from build123d import *

# Parameters (mm, degrees)
SKETCH1_R           = 1.5
SKETCH1_W           = 42
SKETCH1_H           = 20.5
BOSS_EXTRUDE1_DEPTH = 4


with BuildPart() as part:
    # Sketch1 → Boss-Extrude1 (new body)
    with BuildSketch(Plane.XY):
        with BuildLine():
            Line((0, 0), (0, 28))
            Line((0, 28), (-54, 28))
            Line((-54, 28), (-54, 33))
            Line((-54, 33), (-78, 33))
            Line((-78, 33), (-78, 28))
            Line((-78, 28), (-92, 28))
            Line((-92, 28), (-92, 21.4))
            Line((-92, 21.4), (-88, 21.4))
            ThreePointArc((-88, 21.4), (-86, 19.4), (-88, 17.4))
            Line((-88, 17.4), (-92, 17.4))
            Line((-92, 17.4), (-92, 11.6))
            Line((-92, 11.6), (-88, 11.6))
            ThreePointArc((-88, 11.6), (-86, 9.6), (-88, 7.6))
            Line((-88, 7.6), (-92, 7.6))
            Line((-92, 7.6), (-92, 0))
            Line((-92, 0), (0, 0))
        make_face()
        with Locations((-10, 21)):
            Circle(SKETCH1_R, mode=Mode.SUBTRACT)
        with Locations((-10, 6)):
            Circle(SKETCH1_R, mode=Mode.SUBTRACT)
        with Locations((-63, 14.5)):
            Rectangle(SKETCH1_W, SKETCH1_H, mode=Mode.SUBTRACT)
    extrude(amount=BOSS_EXTRUDE1_DEPTH)


solid = part.part
CAD build for the part. Positions are in the model's coordinates, mm. A direction names the side the tool comes from. Coordinates: 2 decimals unless noted, no trailing zeros. Order: outer loops, then holes, each group sorted by start corner. A loop starts at its lowest first (then second) coordinate and runs counter-clockwise, first axis right, second up.
Item 1: Band-saw the part on C-C on z = 2.3. List the corners of the cut face in (x, y).
Check sheet entries:
outline: (-92, 0) - (0, 0) - (0, 28) - (-54, 28) - (-54, 33) - (-78, 33) - (-78, 28) - (-92, 28) - (-92, 21.4) - (-88, 21.4) arc R2 cw to (-88, 17.4) - (-92, 17.4) - (-92, 11.6) - (-88, 11.6) arc R2 cw to (-88, 7.6) - (-92, 7.6) - close; hole (-84, 4.25) - (-42, 4.25) - (-42, 24.75) - (-84, 24.75) - close; hole circle Ø3 at (-10, 6); hole circle Ø3 at (-10, 21)
Item 2: Pin check, flat tips, straight feed: pin 1 Ø1.2 at (x, z) = (-89.5, 2.5) entering from +Y; pin 2 Ø2 at (y, z) = (30.5, 2.5) entering from -X; pin 3 Ø8 at (x, y) = (-69.5, 8.5) entering from -Z; pin 4 Ø2 at (y, z) = (10, 2.5) entering from -X. Stop position of each tip, or through.
Check sheet entries:
pin 1: stops at y = 28
pin 2: stops at x = -78
pin 3: passes through
pin 4: stops at x = -86.57
Item 3: 3-axis set-ups, long thin cutter, end or side, ignore diameter. For faces 1 (the face through (-90, 11.6, 2)), 2 (the face through (-36, 17, 0)), 3 (the face through (-27, 28, 2)), 4 (the face through (-63, 4.25, 2)), 5 (the face through (-78, 31, 2)): which of +Z, -Z, +X, -X, +Y, -Y reach the whole face in a straight line?
Check sheet entries:
face 1: +Z, -Z, -X
face 2: -Z, +X, -X, +Y, -Y
face 3: +Z, -Z, +X, +Y
face 4: +Z, -Z
face 5: +Z, -Z, -X, +Y
Item 4: Band-saw the part on B-B on x = -10. List the corners of the cut face in (y, z), plus the area to 3 significant figures.
Check sheet entries:
outline: (0, 0) - (4.5, 0) - (4.5, 4) - (0, 4) - close; (7.5, 0) - (19.5, 0) - (19.5, 4) - (7.5, 4) - close; (22.5, 0) - (28, 0) - (28, 4) - (22.5, 4) - close
area: 88.0 mm2
Item 5: Drill centre lines: L1, parallel to Y at x = -10, z = 0.65; L2, parallel to Y at x = -44, z = 0.5; L3, parallel to Y at x = -60, z = 1.6. Where is each one in solid material? Low to high.
Check sheet entries:
L1: y = 0 to 4.5, 7.5 to 19.5, 22.5 to 28
L2: y = 0 to 4.25, 24.75 to 28
L3: y = 0 to 4.25, 24.75 to 33
Item 6: Band-saw the part on D-D on x = -81.5. List the corners of the cut face in (y, z), plus the area to 3 significant figures.
Check sheet entries:
outline: (0, 0) - (4.25, 0) - (4.25, 4) - (0, 4) - close; (24.75, 0) - (28, 0) - (28, 4) - (24.75, 4) - close
area: 30.0 mm2
Item 7: Two-plate mould, pull along X, no slides. Class faces 6 (the face through (-11.5, 6.07, 1.97)), 7 (the face through (-92, 25, 2)), 8 (the face through (-90, 21.4, 2)): +X half, -X half, draft (parallel to the pull), parting line (faces both ways), or undercut.
Check sheet entries:
face 6: undercut
face 7: -X half
face 8: draft
Item 8: Band-saw the part on A-A on x = -67. List the corners of the cut face in (y, z).
Check sheet entries:
outline: (0, 0) - (4.25, 0) - (4.25, 4) - (0, 4) - close; (24.75, 0) - (33, 0) - (33, 4) - (24.75, 4) - close
